For this review, take the finished solid that the model builds, in its own axes (mm). A direction names the side the tool comes from. Give positions to 0.01 mm unless a question says otherwise; leave off trailing zeros. Order: outer loops, then holes, each group sorted by start corner. A loop starts at its lowest first (then second) coordinate and runs counter-clockwise, first axis right, second up. Notation, with made-up numbers: (61.25, 17) - (70.25, 17) arc R22 ccw to (70.25, 44) - close; hole circle Ø3 at (84, 27). An arc over 180 degrees is marked (long way). Answer as a JSON object with one key per item and string values. Group by question number.
from build123d import *

# Parameters (mm, degrees)
SKETCH_1_R          = 3.1
EXTRUDE_2_DEPTH     = 5
SKETCH_2_R          = 0.75
CUT_EXTRUDE_1_DEPTH = 5


with BuildPart() as part:
    # 草图1 → 凸台-拉伸2 (new body)
    # profile 1 of 13: a face of its own
    with BuildSketch(Plane.XY):
        with BuildLine():
            ThreePointArc((46.84834221, 57.889935626), (22.328704618, 42.947388438), (21.598208517, 14.242707294))
            Line((21.598208517, 14.242707294), (24.63359588, 15.995189006))
            ThreePointArc((24.63359588, 15.995189006), (25.35979925, 41.197395358), (46.84834221, 54.385310198))
            Line((46.84834221, 54.385310198), (46.84834221, 57.889935626))
        make_face()
    # profile 2 of 13: a face of its own
    with BuildSketch(Plane.XY):
        with BuildLine():
            Line((71.95935283, 15.995189006), (74.994740193, 14.242707294))
            ThreePointArc((74.994740193, 14.242707294), (77.459361516, 20.887435435), (78.296474355, 27.924907455))
            ThreePointArc((78.296474355, 27.924907455), (70.030591529, 48.60407936), (49.787930978, 57.887810471))
            Line((49.787930978, 57.887810471), (49.787930978, 54.382903546))
            ThreePointArc((49.787930978, 54.382903546), (67.554895896, 46.128291749), (74.796474355, 27.924907455))
            ThreePointArc((74.796474355, 27.924907455), (74.077439034, 21.793687331), (71.95935283, 15.995189006))
        make_face()
    # profile 3 of 13: a face of its own
    with BuildSketch(Plane.XY):
        with BuildLine():
            ThreePointArc((23.098208517, 11.644631083), (48.296474355, -2.075092545), (73.494740193, 11.644631083))
            Line((73.494740193, 11.644631083), (70.45935283, 13.397112794))
            ThreePointArc((70.45935283, 13.397112794), (48.296474355, 1.424907455), (26.13359588, 13.397112794))
            Line((26.13359588, 13.397112794), (23.098208517, 11.644631083))
        make_face()
    # profile 4 of 13: a face of its own
    with BuildSketch(Plane.XY):
        with BuildLine():
            ThreePointArc((21.598208517, 14.242707294), (22.315712241, 12.924907455), (23.098208517, 11.644631083))
            Line((23.098208517, 11.644631083), (26.13359588, 13.397112794))
            ThreePointArc((26.13359588, 13.397112794), (25.346801155, 14.674907455), (24.63359588, 15.995189006))
            Line((24.63359588, 15.995189006), (21.598208517, 14.242707294))
        make_face()
    # profile 5 of 13: a face of its own
    with BuildSketch(Plane.XY):
        with BuildLine():
            ThreePointArc((24.63359588, 15.995189006), (25.346801155, 14.674907455), (26.13359588, 13.397112794))
            Line((26.13359588, 13.397112794), (43.925927509, 23.66952025))
            ThreePointArc((43.925927509, 23.66952025), (43.013719392, 24.874907455), (42.425927509, 26.267596461))
            Line((42.425927509, 26.267596461), (24.63359588, 15.995189006))
        make_face()
    # profile 6 of 13: a face of its own
    with BuildSketch(Plane.XY):
        with BuildLine():
            Line((52.565394479, 27.19229608), (54.167021201, 26.267596461))
            ThreePointArc((54.167021201, 26.267596461), (54.338838783, 27.088347762), (54.396474355, 27.924907455))
            ThreePointArc((54.396474355, 27.924907455), (53.108328748, 31.67404833), (49.787930978, 33.839766468))
            Line((49.787930978, 33.839766468), (49.787930978, 32.638782116))
            Line((49.787930978, 32.638782116), (46.84834221, 32.638782116))
            Line((46.84834221, 32.638782116), (46.84834221, 33.850522469))
            ThreePointArc((46.84834221, 33.850522469), (43.027133101, 30.998023585), (42.425927509, 26.267596461))
            Line((42.425927509, 26.267596461), (43.927397053, 27.134470306))
            Line((43.927397053, 27.134470306), (45.427397053, 24.536394095))
            Line((45.427397053, 24.536394095), (43.925927509, 23.66952025))
            ThreePointArc((43.925927509, 23.66952025), (48.296474355, 21.824907455), (52.667021201, 23.66952025))
            Line((52.667021201, 23.66952025), (51.065394479, 24.594219869))
            Line((51.065394479, 24.594219869), (52.565394479, 27.19229608))
        make_face()
        with Locations((48.296474355, 27.924907455)):
            Circle(SKETCH_1_R, mode=Mode.SUBTRACT)
    # profile 7 of 13: a face of its own
    with BuildSketch(Plane.XY):
        with BuildLine():
            ThreePointArc((42.425927509, 26.267596461), (43.013719392, 24.874907455), (43.925927509, 23.66952025))
            Line((43.925927509, 23.66952025), (45.427397053, 24.536394095))
            Line((45.427397053, 24.536394095), (43.927397053, 27.134470306))
            Line((43.927397053, 27.134470306), (42.425927509, 26.267596461))
        make_face()
    # profile 8 of 13: a face of its own
    with BuildSketch(Plane.XY):
        with BuildLine():
            ThreePointArc((52.667021201, 23.66952025), (53.579229318, 24.874907455), (54.167021201, 26.267596461))
            Line((54.167021201, 26.267596461), (52.565394479, 27.19229608))
            Line((52.565394479, 27.19229608), (51.065394479, 24.594219869))
            Line((51.065394479, 24.594219869), (52.667021201, 23.66952025))
        make_face()
    # profile 9 of 13: a face of its own
    with BuildSketch(Plane.XY):
        with BuildLine():
            Line((49.787930978, 32.638782116), (49.787930978, 33.839766468))
            ThreePointArc((49.787930978, 33.839766468), (48.3187942, 34.024866621), (46.84834221, 33.850522469))
            Line((46.84834221, 33.850522469), (46.84834221, 32.638782116))
            Line((46.84834221, 32.638782116), (49.787930978, 32.638782116))
        make_face()
    # profile 10 of 13: a face of its own
    with BuildSketch(Plane.XY):
        with BuildLine():
            Line((49.787930978, 33.839766468), (49.787930978, 54.382903546))
            ThreePointArc((49.787930978, 54.382903546), (48.31816999, 54.424898574), (46.84834221, 54.385310198))
            Line((46.84834221, 54.385310198), (46.84834221, 33.850522469))
            ThreePointArc((46.84834221, 33.850522469), (48.3187942, 34.024866621), (49.787930978, 33.839766468))
        make_face()
    # profile 11 of 13: a face of its own
    with BuildSketch(Plane.XY):
        with BuildLine():
            ThreePointArc((70.45935283, 13.397112794), (71.246147555, 14.674907455), (71.95935283, 15.995189006))
            Line((71.95935283, 15.995189006), (54.167021201, 26.267596461))
            ThreePointArc((54.167021201, 26.267596461), (53.579229318, 24.874907455), (52.667021201, 23.66952025))
            Line((52.667021201, 23.66952025), (70.45935283, 13.397112794))
        make_face()
    # profile 12 of 13: a face of its own
    with BuildSketch(Plane.XY):
        with BuildLine():
            ThreePointArc((73.494740193, 11.644631083), (74.277236468, 12.924907455), (74.994740193, 14.242707294))
            Line((74.994740193, 14.242707294), (71.95935283, 15.995189006))
            ThreePointArc((71.95935283, 15.995189006), (71.246147555, 14.674907455), (70.45935283, 13.397112794))
            Line((70.45935283, 13.397112794), (73.494740193, 11.644631083))
        make_face()
    # profile 13 of 13: a face of its own
    with BuildSketch(Plane.XY):
        with BuildLine():
            Line((49.787930978, 54.382903546), (49.787930978, 57.887810471))
            ThreePointArc((49.787930978, 57.887810471), (48.318162639, 57.924899616), (46.84834221, 57.889935626))
            Line((46.84834221, 57.889935626), (46.84834221, 54.385310198))
            ThreePointArc((46.84834221, 54.385310198), (48.31816999, 54.424898574), (49.787930978, 54.382903546))
        make_face()
    extrude(amount=EXTRUDE_2_DEPTH)

    # 草图2 → 切除-拉伸1 (cut)
    with BuildSketch(Plane.XY.offset(5)):
        with Locations((23.614750347, 42.174907455)):
            Circle(SKETCH_2_R)
        with Locations((72.978198363, 42.174907455)):
            Circle(SKETCH_2_R)
        with Locations((48.296474355, -0.575092545)):
            Circle(SKETCH_2_R)
    extrude(amount=-CUT_EXTRUDE_1_DEPTH, mode=Mode.SUBTRACT)


solid = part.part
1) Consider section C-C (z = 4.05). Give the boundary of the cut face in (x, y), plus the area to 3 significant figures.
2) Consider section D-D (y = 32). Give the boundary of the cut face in (x, z), plus the area to 3 significant figures.
3) Consider section B-B (y = 10). Give the boundary of the cut face in (x, z).
4) Mouldability with a two-part tool opening along X and no side actions: class faces 3 (the face through (46.848, 44, 2)), 4 (the face through (48, 24, 5)) as released by +X, released by -X, zero draft, split by the parting line, or undercut.
5) For pin 1 (2.5 mm diameter, centred on x = 72.98, y = 42.17, fed in from -Z); pin 2 (1.4 mm diameter, centred on x = 48.3, y = -0.58, fed in from +Z); pin 3 (2.5 mm diameter, centred on y = 46.5, z = 3.5, fed in from +X); pin 4 (1.5 mm diameter, centred on x = 69.5, z = 0.5, fed in from -Y), all flat-tipped, find the tip position at first contact; note any pin that passes through.
6) Consider section A-A (x = 32). Give the boundary of the cut face in (y, z), plus the area to 3 significant figures.
7) For faces 1 (the face through (48.228, 21.825, 2.465)), 2 (the face through (48, 24, 0)), list the 3-axis set-ups (+Z, -Z, +X, -X, +Y, -Y) from which the entire face can be reached by the end or side of a thin tool; tool diameter is ignored.
8) For line 1 (X direction, y = 38.5, z = 4.2); line 2 (Y direction, x = 68, z = 4.35); line 3 (Y direction, x = 44, z = 2.5), list the stretches that pass through material, from the lowest coordinate up.
Result set:
{
 "1": {"outline": "circle Ø60 at (48.3, 27.92); hole circle Ø1.5 at (23.61, 42.17); hole (24.63, 16) - (42.43, 26.27) arc R6.1 cw to (46.85, 33.85) - (46.85, 54.39) arc R26.5 ccw to start; hole (26.13, 13.4) arc R26.5 ccw to (70.46, 13.4) - (52.67, 23.67) arc R6.1 cw to (43.93, 23.67) - close; hole circle Ø6.2 at (48.3, 27.92); hole circle Ø1.5 at (48.3, -0.58); hole (49.79, 33.84) arc R6.1 cw to (54.17, 26.27) - (71.96, 16) arc R26.5 ccw to (49.79, 54.38) - close; hole circle Ø1.5 at (72.98, 42.17)", "area": "885 mm2"},
 "2": {"outline": "(18.57, 0) - (22.11, 0) - (22.11, 5) - (18.57, 5) - close; (43.76, 0) - (52.84, 0) - (52.84, 5) - (43.76, 5) - close; (74.48, 0) - (78.02, 0) - (78.02, 5) - (74.48, 5) - close", "area": "80.8 mm2"},
 "3": {"outline": "(24.24, 0) - (28.78, 0) - (28.78, 5) - (24.24, 5) - close; (67.81, 0) - (72.35, 0) - (72.35, 5) - (67.81, 5) - close"},
 "4": {"face 3": "undercut", "face 4": "zero draft"},
 "5": {"pin 1": "stops at z = 0", "pin 2": "passes through", "pin 3": "stops at x = 72.79", "pin 4": "stops at y = 5.98"},
 "6": {"outline": "(2.74, 0) - (7.03, 0) - (7.03, 5) - (2.74, 5) - close; (16.78, 0) - (20.25, 0) - (20.25, 5) - (16.78, 5) - close; (48.82, 0) - (53.11, 0) - (53.11, 5) - (48.82, 5) - close", "area": "60.2 mm2"},
 "7": {"face 1": "+Z, -Z", "face 2": "-Z, +X, -X, +Y, -Y"},
 "8": {"line 1": "x = 20.22 to 24, 46.85 to 49.79, 72.59 to 76.37", "line 2": "y = 5.3 to 10.2, 14.82 to 18.28, 45.65 to 50.55", "line 3": "y = -1.77 to 1.78, 23.59 to 32.26, 54.07 to 57.62"}
}
